For this review, use the dimensioned drawing (mm, ordinates from the lowest corner) and the shaded views. A direction names the side the tool comes from. Give positions to 0.01 mm unless a question says otherwise; leave off trailing zeros. Write each loop counter-clockwise with the first axis right and the second up, starting at its lowest first coordinate (ties: lowest second). Pieces come first, ordered by that corner, then holes. Notation, with made-up numbers: (22.5, 26) -> (78.5, 26) arc R22 cw to (78.5, 45) -> close; hole circle Ø8 at (-35.75, 85.5). An arc over 180 degrees is marked (long way). Write each question's results on one line, items separated by ' | '. Start each with the question number.
(1) For the marked faces 1 and 2, list the 3-axis set-ups (+Z, -Z, +X, -X, +Y, -Y) from which the entire face can be reached by the end or side of a thin tool; tool diameter is ignored.
(2) Clearance check with flat-ended pins moving along their axes: pin 1 (15 mm diameter, centred on x = 179.39, y = 25.4, fed in from +Z); pin 2 (8.5 mm diameter, centred on x = 23.81, y = 25.4, fed in from +Z); pin 3 (5 mm diameter, centred on x = 133, y = 129.5, fed in from -Z). State where each tip first meets the part, or that it passes through.
(3) Take a section at B-B (x = 101.6). State the section outline as (y, z) points.
(4) Take a section at D-D (z = 218). State the section outline as (x, y) points.
(5) To check wall thickness, follow probe 1 along X at (y, z) = (177, 13); probe 2 along Z at (x, y) = (120, 145); probe 3 along Y at (x, z) = (90, 75.5) (1 decimal). State the ranges of each line that lie inside material, in increasing order.
(6) Take a section at C-C (y = 156). State the section outline as (x, z) points.
(7) Take a section at A-A (y = 25.4). Count the separate pieces of the cut face and the enclosed holes in it, plus the area to 3 significant figures.
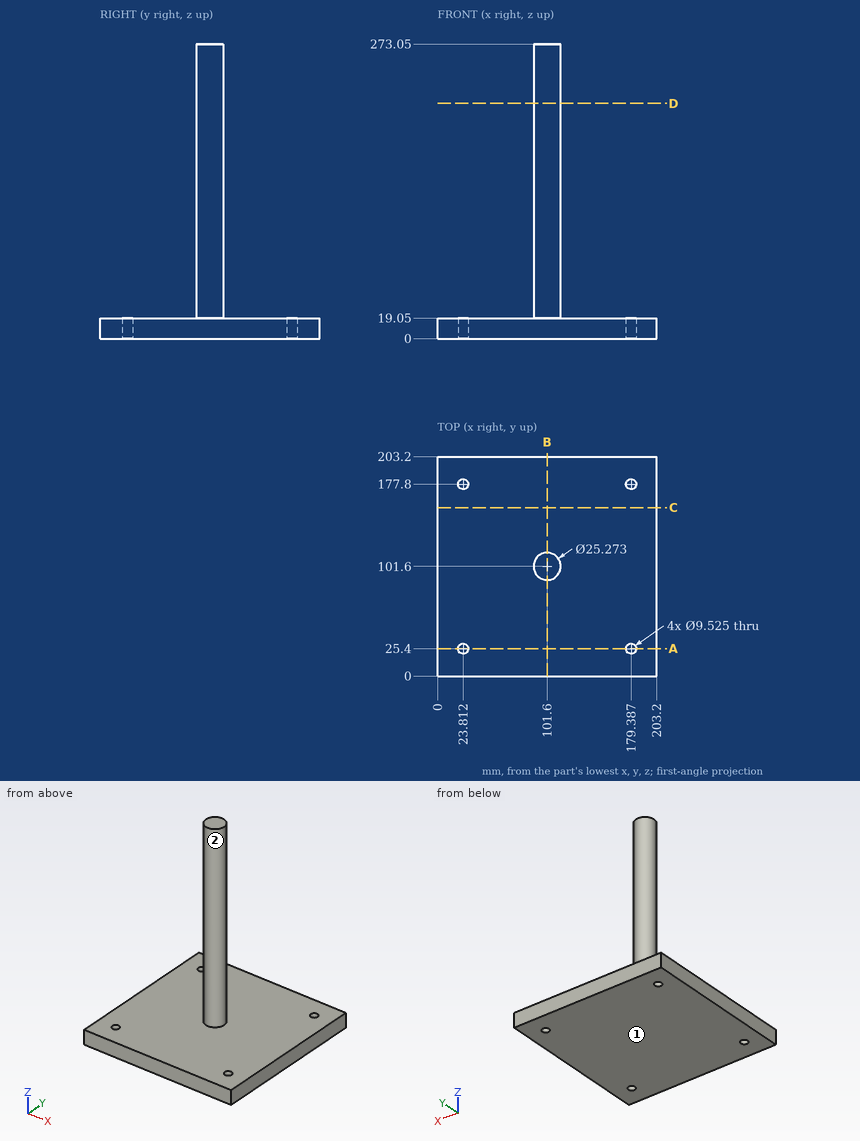
Report:
1) face 1: -Z, +X, -X, +Y, -Y | face 2: +Z
2) pin 1: z = 19.05 | pin 2: through | pin 3: z = 0
3) outline: (0, 0) -> (203.2, 0) -> (203.2, 19.05) -> (114.24, 19.05) -> (114.24, 273.05) -> (88.96, 273.05) -> (88.96, 19.05) -> (0, 19.05) -> close
4) outline: circle Ø25.27 at (101.6, 101.6)
5) probe 1: 0 to 19.12, 28.51 to 174.69, 184.08 to 203.2 | probe 2: 0 to 19.05 | probe 3: 96.6 to 106.6
6) outline: (0, 0) -> (203.2, 0) -> (203.2, 19.05) -> (0, 19.05) -> close
7) separate pieces: 3 | enclosed holes: 0 | area: 3,510 mm2
